Verification items for the finished model (mm, model axes). A direction names the side the tool comes from. Give positions to 0.01 mm unless a question says otherwise; leave off trailing zeros. Loops run counter-clockwise (first coordinate to the right, second up) from the corner with the lowest first, then second, coordinate; pieces in that order, holes last. Notation, with made-up numbers: M 10,24.5 L 56,24.5 A13 ccw 56,49.5 Z; hole C 12.25,77 d6. An arc over 180 degrees is marked long. Put each result on its own line as item: value. Start each with the question number.
from build123d import *

# Parameters (mm, degrees)
F2_W     = 11
F2_H     = 12
F3_DEPTH = 40
F4_SIZE  = 1
F5_W     = 2.5
F5_H     = 0.6369768083
F5_W_2   = 2.8
F5_H_2   = 0.9896519035


with BuildPart() as f1:
    # F0 (on Front) → F1 (revolve)
    with BuildSketch(Plane.XZ):
        with BuildLine():
            Line((0, 15), (0, 9))
            Line((0, 9), (30, 9))
            Line((30, 9), (30, 35))
            Line((30, 35), (17.5, 35))
            ThreePointArc((17.5, 35), (15.732233047, 34.267766953), (15, 32.5))
            Line((15, 32.5), (15, 20))
            ThreePointArc((15, 20), (13.5355339059, 16.4644660941), (10, 15))
            Line((10, 15), (0, 15))
        make_face()
    revolve(axis=Axis((13.2997054259, 0, 0), (1, 0, 0)))

    # F2 (on Front) → F3 (cut, symmetric)
    with BuildSketch(Plane.XZ):
        with Locations((24.5, 0)):
            Rectangle(F2_W, F2_H)
    extrude(amount=F3_DEPTH, both=True, mode=Mode.SUBTRACT)

    # F4
    f4_edges = [f1.edges().sort_by_distance(p)[0] for p in [
        (0, 0, -9),
        (30, 20.595042, 6),
        (30, -20.595042, 6),
        (30, -20.595042, -6),
        (30, 20.595042, -6),
    ]]
    chamfer(f4_edges, length=F4_SIZE)

    # F5 (on Front) → F6 (revolve, cut)
    with BuildSketch(Plane.XZ):
        with Locations((7.25, -15.3184884042)):
            Rectangle(F5_W, F5_H)
        Polygon((6, -15), (8.5, -15), (8.8, 15), (6, 15), align=None)
        with Locations((7.4, 15.4948259518)):
            Rectangle(F5_W_2, F5_H_2)
    revolve(axis=Axis((6, 0, -0.3860071301), (0, 0, -1)), mode=Mode.SUBTRACT)


solid = f1.part
Q1. Release check for a two-part mould opening along Y. For faces 1 (the face through (4.93, -4.506, 14.307)), 2 (the face through (8.64, -0.83, 11.83)), 3 (the face through (3.47, -0.11, -11.77)), 4 (the face through (30, 0, 18)) record: pulls with the +Y half, pulls with the -Y half, needs draft (parallel to the pull), parting line crosses it, or undercut.
Q2. Cross-section at C-C, the plane y = 0. State how many separate pieces and enclosed holes the cut face has, then the cut area to 3 significant figures.
Q3. Cross-section at B-B, the plane x = 14. Record the boundary of the cut face in (y, z).
Q4. Go/stop test with flat-tipped pins: pin 1 (5 mm diameter, centred on x = 13.5, z = -26, fed in from -Y); pin 2 (10 mm diameter, centred on x = 26, z = 2.5, fed in from +Y); pin 3 (10 mm diameter, centred on y = -4.5, z = -4.5, fed in from +X); pin 4 (6 mm diameter, centred on y = 25, z = 2.5, fed in from +X). Record where each tip stops, or that it passes through.
Q5. Scan lines: L1, parallel to Z at x = 9, y = 0; L2, parallel to Z at x = 18.5, y = 0; L3, parallel to X at y = -12, z = -20. Record each from-to range of solid material in increasing order.
Q6. Set-up check for faces 5 (the face through (16, 0, -9)), 6 (the face through (24, 20, 6)), 7 (the face through (15, -15, 14)): record each of +Z, -Z, +X, -X, +Y, -Y from which the full face is reachable in a straight line by a thin tool's end or side.
Q7. Cross-section at A-A, the plane z = 0. Record the boundary of the cut face in (x, y), then the cut area to 3 significant figures.
Ans:
1. face 1: parting line crosses it
1. face 2: undercut
1. face 3: undercut
1. face 4: needs draft
2. separate pieces: 4
2. enclosed holes: 0
2. area: 903 mm^2
3. outline: C 0,0 d34; hole C 0,0 d18
4. pin 1: stops at y = -23.61
4. pin 2: stops at y = 34.48
4. pin 3: stops at x = 30
4. pin 4: stops at x = 19
5. L1: z = -15 to -9, 9 to 15
5. L2: z = -35 to -9, 9 to 35
5. L3: x = 15 to 30
6. face 5: +X, -X
6. face 6: +X, +Y, -Y
6. face 7: -X
7. outline: M 0,-15 L 10,-15 A5 cw 15,-20 L 15,-32.5 A2.5 ccw 17.5,-35 L 19,-35 L 19,-9 L 1,-9 L 0,-10 Z; M 0,10 L 1,9 L 19,9 L 19,35 L 17.5,35 A2.5 ccw 15,32.5 L 15,20 A5 cw 10,15 L 0,15 Z
7. area: 395 mm^2
